from build123d import *

# Parameters (mm, degrees)
SKETCH2_W           = 85.14
SKETCH2_H           = 63.86
SKETCH2_R           = 1.5
BOSS_EXTRUDE1_DEPTH = 0.825
FILLET1_R           = 3
CHAMFER1_SIZE       = 3


with BuildPart() as part:
    # Sketch2 → Boss-Extrude1 (new body, symmetric)
    with BuildSketch(Plane(origin=(0, 0, 0), x_dir=(1, 0, 0), z_dir=(0, 1, 0))):
        Rectangle(SKETCH2_W, SKETCH2_H)
        with Locations((-19.11, 20.91)):
            Circle(SKETCH2_R, mode=Mode.SUBTRACT)
        with Locations((39.01, 20.91)):
            Circle(SKETCH2_R, mode=Mode.SUBTRACT)
        with Locations((39.01, -28.43)):
            Circle(SKETCH2_R, mode=Mode.SUBTRACT)
        with Locations((-19.11, -28.43)):
            Circle(SKETCH2_R, mode=Mode.SUBTRACT)
    extrude(amount=BOSS_EXTRUDE1_DEPTH, both=True)

    # Fillet1
    fillet1_edges = [part.edges().sort_by_distance(p)[0] for p in [
        (42.57, 0, 31.93),
        (-42.57, 0, 31.93),
        (-42.57, 0, -31.93),
    ]]
    fillet(fillet1_edges, radius=FILLET1_R)

    # Chamfer1
    chamfer1_edges = [part.edges().sort_by_distance(p)[0] for p in [
        (42.57, 0, -31.93),
    ]]
    chamfer(chamfer1_edges, length=CHAMFER1_SIZE)


solid = part.part
Read the model definition and answer for the solid it produces. Units are mm, in the model's axes. Coordinates: 2 decimals unless noted, no trailing zeros. Order: outer loops, then holes, each group sorted by start corner. A loop starts at its lowest first (then second) coordinate and runs counter-clockwise, first axis right, second up. Notation, with made-up numbers: M 23,19.5 L 76,19.5 A18 cw 76,35.5 Z; hole C 65.25,20.25 d3. An arc over 180 degrees is marked long. Put each result on its own line as item: value. Start each with the question number.
Item 1: The mould has two halves that part along Z. Classify faces 1 (the face through (40.44, -0.01, 27.98)), 2 (the face through (41.71, 0.01, 31.03)), 3 (the face through (42.57, 0, 0)): +Z half, -Z half, draft (parallel to the pull), parting line (faces both ways), or undercut.
Item 2: Section A-A, the plane x = -19.11 is taken. Determine the outline of the cut face in (y, z) (3 decimals).
Item 3: Consider probe 1 along X at (y, z) = (0.25, 28.43); probe 2 along Z at (x, y) = (39.01, -0.05); probe 3 along X at (y, z) = (-0.15, -21.5). Determine where each line is inside the solid, lowest interval first. Write a range as [from, to].
Item 4: Section B-B, the plane z = -20.91 is taken. Determine the outline of the cut face in (x, y) (3 decimals).
Computed:
1. face 1: undercut
1. face 2: +Z half
1. face 3: draft
2. outline: M -0.825,-31.93 L 0.825,-31.93 L 0.825,-22.41 L -0.825,-22.41 Z; M -0.825,-19.41 L 0.825,-19.41 L 0.825,26.93 L -0.825,26.93 Z; M -0.825,29.93 L 0.825,29.93 L 0.825,31.93 L -0.825,31.93 Z
3. probe 1: x = [-42.57, -20.61], [-17.61, 37.51], [40.51, 42.57]
3. probe 2: z = [-31.93, -22.41], [-19.41, 26.93], [29.93, 31.93]
3. probe 3: x = [-42.57, -20.49], [-17.73, 37.63], [40.39, 42.57]
4. outline: M -42.57,-0.825 L -20.61,-0.825 L -20.61,0.825 L -42.57,0.825 Z; M -17.61,-0.825 L 37.51,-0.825 L 37.51,0.825 L -17.61,0.825 Z; M 40.51,-0.825 L 42.57,-0.825 L 42.57,0.825 L 40.51,0.825 Z
